The model under review builds one solid part; all positions refer to its coordinate system, in mm. A direction names the side the tool comes from. Round coordinates to 2 decimals unless told otherwise and drop trailing zeros. Loops run counter-clockwise (first coordinate to the right, second up) from the corner with the lowest first, then second, coordinate; pieces in that order, holes last. Notation, with made-up numbers: M 7.5,89.25 L 22.5,89.25 A27 ccw 22.5,125.25 Z; hole C -22,6 d2. An arc over 180 degrees is marked long. Answer as a JSON object with one key per item and string values. Group by question number.
Item 1: Consider section C-C (y = 2.54). Give the boundary of the cut face in (x, z) (1 decimal), and give its area (3 significant figures).
Item 2: Tool access review of faces 5 (the face through (2.461, 2.318, 4.732)), 6 (the face through (14.414, 3, 0)), 7 (the face through (-14.414, 3, 0)), 8 (the face through (1.116, 1.323, -15.638)), 9 (the face through (-0.07, 0.89, 15.64)): name each direction out of +Z, -Z, +X, -X, +Y, -Y from which nothing blocks a thin tool from reaching the whole face with its end or side.
Item 3: Insertion check: P1, Ø1.7, axis at y = 2, z = -0.5, coming from the -X side; P2, Ø1, axis at x = 2, y = 2, coming from the -Z side; P3, Ø2.5, axis at x = 0, y = 2.54, coming from the +Z side. Each pin has a flat end and moves straight along its axis. Give the tip position at first contact, or say it passes through.
Item 4: To check wall thickness, follow line 1 (X direction, y = 7, z = 0) (1 decimal); line 2 (X direction, y = 3.6, z = 0); line 3 (Y direction, x = 15.1, z = 0). State the ranges of each line that lie inside material, in increasing order.
Item 5: The part is to be moulded in two halves that separate along Z. For faces 1 (the face through (-7, 4.572, 0)), 2 (the face through (0, 3, 14.414)), 3 (the face through (-3.441, 6.826, -15.497)), 4 (the face through (1.11, 5.52, 16.79)), say which applies: +Z half, -Z half, draft (parallel to the pull), parting line (faces both ways), or undercut.
Autodesk Inventor part; units mm, degrees
ref_plane "Work Plane1" through (-16.8275, 0, 0) normal (1, 0, 0) x (0, 1, 0)
ref_plane "XZ Plane" through (0, 0, 0) normal (0, 1, 0) x (-1, 0, 0)
ref_plane "XY Plane" through (0, 0, 0) normal (0, 0, 1) x (1, 0, 0)
sketch "Sketch1" plane through (0, 0, 0) normal (0, 1, 0) x (-1, 0, 0)
  circle A0 centre (0, 0) radius 16.8275
  dimension "d0" = 33.655
extrude "Extrusion1" add sketch "Sketch1" along normal blind 4.572
sketch "Sketch2" plane through (0, 4.572, 0) normal (0, 1, 0) x (1, 0, 0)
  circle A0 centre (0, 0) radius 15.875
  circle A1 centre (0, 0) radius 16.8275
  dimension "d3" = 31.75
extrude "Extrusion2" add sketch "Sketch2" along normal blind 4.572
ref_plane "Work Plane1" through (-16.8275, 0, 0) normal (1, 0, 0) x (0, 1, 0)
sketch "Sketch3" plane through (-16.8275, 0, 0) normal (1, 0, 0) x (0, 1, 0)
  circle A0 centre (2.54, 0) radius 1.651
  line L0 (0, 16.8275) -> (0, -16.8275)
  point P0 (0, 0)
  dimension "d6" = 3.302
  dimension "d7" = 2.54
extrude "Extrusion3" cut sketch "Sketch3" along normal blind 2.413
pattern_circular "Circular Pattern1" count 4 over 360 about axis through (0, 0, 0) along (0, 1, 0) of "Extrusion3"
sketch "Sketch4" plane through (0, 4.572, 0) normal (0, 1, 0) x (1, 0, 0)
  circle A0 centre (0, 0) radius 5.334
  dimension "d13" = 10.668
extrude "Extrusion4" cut sketch "Sketch4" against normal blind 25.4
properties part number "BallastThrustWasherSpacer" material "ABS Plastic"
Geometry results:
{
 "1": {"outline": "M -16.7,-1.7 A16.8 ccw -1.7,-16.7 L -1.7,-14.4 L 1.7,-14.4 L 1.7,-16.7 A16.8 ccw 16.7,-1.7 L 14.4,-1.7 L 14.4,1.7 L 16.7,1.7 A16.8 ccw 1.7,16.7 L 1.7,14.4 L -1.7,14.4 L -1.7,16.7 A16.8 ccw -16.7,1.7 L -14.4,1.7 L -14.4,-1.7 Z; hole C 0,0 d10.7", "area": "769 mm^2"},
 "2": {"face 5": "+Y, -Y", "face 6": "+X", "face 7": "-X", "face 8": "-Z", "face 9": "+Z"},
 "3": {"P1": "stops at x = -14.41", "P2": "stops at z = -16.76", "P3": "stops at z = 14.41"},
 "4": {"line 1": "x = -16.8 to -15.9, 15.9 to 16.8", "line 2": "x = -14.41 to -5.33, 5.33 to 14.41", "line 3": "y = 0 to 0.89, 4.19 to 4.57"},
 "5": {"face 1": "undercut", "face 2": "+Z half", "face 3": "undercut", "face 4": "parting line"}
}
